Source: CAD feature listing. Evaluate the final solid. Frame: model axes, mm. Face numbers are marked on the shaded views. A direction names the side the tool comes from. Coordinates: 2 decimals unless noted, no trailing zeros. Write each loop counter-clockwise with the first axis right and the second up, starting at its lowest first coordinate (ties: lowest second). Pieces come first, ordered by that corner, then holes. Notation, with made-up numbers: M 17,50.25 L 37,50.25 A35 cw 37,85.25 Z; hole C 47.25,-28.75 d7. An arc over 180 degrees is marked long. Answer as CSV lines item,"result". Start each with the question number.
1. Contact query for a flat-ended pin moving along its axis: pin 1 Ø0.8 at (x, z) = (-4, 2) entering from -Y. Output: stop coordinate, or through.
2. Section C-C on z = 1.1. Return the cut outline in (x, y), plus the area to 3 significant figures.
3. Section B-B on y = 15.8. Return the cut outline in (x, z), plus the area to 3 significant figures.
4. Section A-A on x = -9.7. Return the cut outline in (y, z).
5. Reachability of the marked faces 4, 5 and 6 from +Z, -Z, +X, -X, +Y, -Y: full face, straight path, thin tool, end or side. Return the list, or none.
6. Mould query, pull axis X, two halves, no side actions, for the marked faces 1, 2 and 3. Classes: pulls with the +X half, pulls with the -X half, needs draft (parallel to the pull), parting line crosses it, or undercut.
7. Line query: probe 1 along Y at (x, z) = (1, 0.7); probe 2 along X at (y, z) = (3.75, 0.3); probe 3 along Y at (x, z) = (-9.75, 2.55). Output: solid intervals per line, ascending. Write a range as [from, to].
8. Section D-D on y = 5. Return the cut outline in (x, z), plus the area to 3 significant figures.
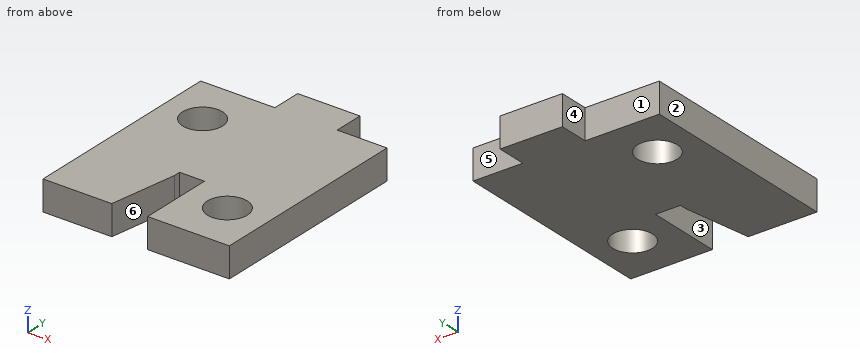
```python
from build123d import *

# Parameters (mm, degrees)
BOSS_EXTRUDE1_DEPTH          = 3
SKETCH2_W                    = 7.45
SKETCH2_H                    = 3
CUT_EXTRUDE1_DEPTH           = 3
SKETCH3_W                    = 3
SKETCH3_H                    = 20.8
BOSS_EXTRUDE2_DEPTH          = 5
CUT_EXTRUDE2_REACH           = 5
F_4_0_4_DIAMETER_HOLE1_D     = 4
F_4_0_4_DIAMETER_HOLE1_DEPTH = 3


with BuildPart() as part:
    # Sketch1 → Boss-Extrude1 (new body)
    with BuildSketch(Plane.XY):
        Polygon((-13.7, 0), (-5.7, 0), (-5.7, 7.5), (-3.2, 7.5), (-3.2, 0), (0, 0), (0, 23.8), (-13.7, 23.8), align=None)
    extrude(amount=BOSS_EXTRUDE1_DEPTH)

    # Sketch2 → Cut-Extrude1 (cut)
    with BuildSketch(Plane.XY.offset(3)):
        with Locations((-9.975, 22.3)):
            Rectangle(SKETCH2_W, SKETCH2_H)
    extrude(amount=-CUT_EXTRUDE1_DEPTH, mode=Mode.SUBTRACT)

    # Sketch3 → Boss-Extrude2 (add)
    with BuildSketch(Plane(origin=(0, 0, 0), x_dir=(0, 0, -1), z_dir=(1, 0, 0))):
        with Locations((-1.5, 10.4)):
            Rectangle(SKETCH3_W, SKETCH3_H)
    extrude(amount=BOSS_EXTRUDE2_DEPTH)

    # Sketch4 → Cut-Extrude2 (cut, up to next)
    with BuildSketch(Plane.XY.offset(3), mode=Mode.PRIVATE) as cut_extrude2_sk1:
        Polygon((-5.7, 0), (-6.8, 0), (-5.7, 6.8), align=None)
    cut_extrude2_tool1 = extrude(cut_extrude2_sk1.sketch, amount=-CUT_EXTRUDE2_REACH, mode=Mode.PRIVATE) & part.part
    add(cut_extrude2_tool1.solids().sort_by_distance((-6.066667, 2.266667, 3))[0], mode=Mode.SUBTRACT)

    # Ø4.0 (4) Diameter Hole1
    with Locations(Plane.XY.offset(3)):
        with Locations((-9.7, 15.8), (1, 5)):
            Hole(F_4_0_4_DIAMETER_HOLE1_D / 2, depth=F_4_0_4_DIAMETER_HOLE1_DEPTH)


solid = part.part
```
Values:
1,pin 1,"y = 7.5"
2,outline,"M -13.7,0 L -6.8,0 L -5.7,6.8 L -5.7,7.5 L -3.2,7.5 L -3.2,0 L 5,0 L 5,20.8 L 0,20.8 L 0,23.8 L -6.25,23.8 L -6.25,20.8 L -13.7,20.8 Z; hole C -9.7,15.8 d4; hole C 1,5 d4"
2,area,"360 mm²"
3,outline,"M -13.7,0 L -11.7,0 L -11.7,3 L -13.7,3 Z; M -7.7,0 L 5,0 L 5,3 L -7.7,3 Z"
3,area,"44.1 mm²"
4,outline,"M 0,0 L 13.8,0 L 13.8,3 L 0,3 Z; M 17.8,0 L 20.8,0 L 20.8,3 L 17.8,3 Z"
5,face 4,"+Z, -Z, -X, +Y"
5,face 5,"+Z, -Z, +X, +Y"
5,face 6,"+Z, -Z, -Y"
6,face 1,"needs draft"
6,face 2,"pulls with the -X half"
6,face 3,"undercut"
7,probe 1,"[0, 3], [7, 20.8]"
7,probe 2,"[-13.7, -6.19], [-3.2, -0.56], [2.56, 5]"
7,probe 3,"[0, 13.8], [17.8, 20.8]"
8,outline,"M -13.7,0 L -5.99,0 L -5.99,3 L -13.7,3 Z; M -3.2,0 L -1,0 L -1,3 L -3.2,3 Z; M 3,0 L 5,0 L 5,3 L 3,3 Z"
8,area,"35.7 mm²"
